from build123d import *

# Parameters (mm, degrees)
F0_W     = 30
F0_H     = 30
F0_R     = 1
F1_DEPTH = 1
F2_W     = 30
F2_H     = 27
F2_R     = 1
F3_DEPTH = 1


with BuildPart() as f1:
    # F0 (on Top) → F1 (new body)
    with BuildSketch(Plane.XY):
        Rectangle(F0_W, F0_H)
        with Locations((-12.5, -12.5)):
            Circle(F0_R, mode=Mode.SUBTRACT)
        with Locations((12.5, -12.5)):
            Circle(F0_R, mode=Mode.SUBTRACT)
        with Locations((-12.5, 12.5)):
            Circle(F0_R, mode=Mode.SUBTRACT)
        with Locations((12.5, 12.5)):
            Circle(F0_R, mode=Mode.SUBTRACT)
    extrude(amount=F1_DEPTH)

    # F2 (on face) → F3 (join)
    with BuildSketch(Plane(origin=(0, 15, 0), x_dir=(-1, 0, 0), z_dir=(0, 1, 0))):
        with Locations((0, -12.5)):
            Rectangle(F2_W, F2_H)
        with Locations((0, -14)):
            Circle(F2_R, mode=Mode.SUBTRACT)
    extrude(amount=F3_DEPTH)


solid = f1.part
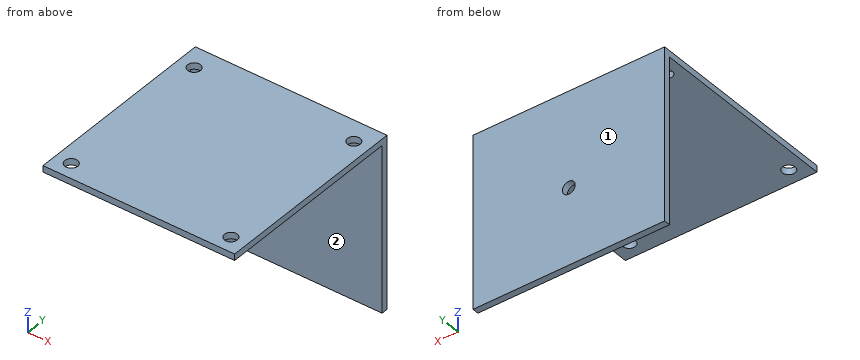
Can you work these out from the model? Positions are in its coordinate system, mm. Face numbers are marked on the shaded views. A direction names the side the tool comes from. Coordinates: 2 decimals unless noted, no trailing zeros. Write each loop counter-clockwise with the first axis right and the second up, starting at its lowest first coordinate (ties: lowest second). Pieces come first, ordered by that corner, then holes. Notation, with made-up numbers: (75, 88) -> (106, 88) arc R23 cw to (106, 106) -> close; hole circle Ø10 at (8, -19.5). An arc over 180 degrees is marked (long way). Write each question's results on one line, items separated by ' | '. Start each with the question number.
Q1. Imagine slicing it at B-B (y = -12.5). Write out the boundary of the cut face in (x, z), then the cut area to 3 significant figures.
Q2. I'm going to push flat-ended pins straight in: pin 1 (6 mm diameter, centred on x = -2.5, z = -7, fed in from -Y); pin 2 (15 mm diameter, centred on x = 0.5, y = 2.5, fed in from -Z). Where does each tip first touch, or does it pass through?
Q3. Imagine slicing it at C-C (z = -14). Write out the boundary of the cut face in (x, y), then the cut area to 3 significant figures.
Q4. If I drill on probe 1 along Y at (x, z) = (-12.5, 0.4); probe 2 along Z at (x, y) = (0, 15.35); probe 3 along Z at (x, y) = (8.5, 4), over which ranges is the centre line in solid material (lowest first)?
Q5. On a 3-axis mill with a long thin cutter (end or side, diameter ignored), from which of +Z, -Z, +X, -X, +Y, -Y can I reach the whole of each face in a straight line? I mean the marked faces 1 and 2. Say none if no direction works.
Q6. Imagine slicing it at A-A (x = -12.5). Write out the boundary of the cut face in (y, z), then the cut area to 3 significant figures.
Q7. Imagine slicing it at D-D (x = 0). Write out the boundary of the cut face in (y, z), then the cut area to 3 significant figures.
Taken from the geometry:
1) outline: (-15, 0) -> (-13.5, 0) -> (-13.5, 1) -> (-15, 1) -> close; (-11.5, 0) -> (11.5, 0) -> (11.5, 1) -> (-11.5, 1) -> close; (13.5, 0) -> (15, 0) -> (15, 1) -> (13.5, 1) -> close | area: 26.0 mm^2
2) pin 1: stops at y = 15 | pin 2: stops at z = 0
3) outline: (-15, 15) -> (-1, 15) -> (-1, 16) -> (-15, 16) -> close; (1, 15) -> (15, 15) -> (15, 16) -> (1, 16) -> close | area: 28.0 mm^2
4) probe 1: y = -15 to -13.5, -11.5 to 11.5, 13.5 to 16 | probe 2: z = -26 to -15, -13 to 1 | probe 3: z = 0 to 1
5) face 1: +Z, -Z, +X, -X, +Y | face 2: -Z, +X, -X, -Y
6) outline: (-15, 0) -> (-13.5, 0) -> (-13.5, 1) -> (-15, 1) -> close; (-11.5, 0) -> (11.5, 0) -> (11.5, 1) -> (-11.5, 1) -> close; (13.5, 0) -> (15, 0) -> (15, -26) -> (16, -26) -> (16, 1) -> (13.5, 1) -> close | area: 53.0 mm^2
7) outline: (-15, 0) -> (15, 0) -> (15, -13) -> (16, -13) -> (16, 1) -> (-15, 1) -> close; (15, -26) -> (16, -26) -> (16, -15) -> (15, -15) -> close | area: 55.0 mm^2
